Could you check a few things on this model? Use its own coordinates, in mm. Coordinates: 2 decimals unless noted, no trailing zeros. Order: outer loops, then holes, each group sorted by start corner. A loop starts at its lowest first (then second) coordinate and runs counter-clockwise, first axis right, second up. Notation, with made-up numbers: (82, 29) -> (113, 29) arc R8 cw to (113, 39) -> close; hole circle Ø5 at (-19.75, -9). An arc over 180 degrees is marked (long way). Use a Markdown table: item, result. Add a question column.
1) If we section it at C-C (y = 1.75): Write out the boundary of the cut face in (x, z), plus the area to 3 significant figures.
2) Will these pins go through, and if not, where does the flat tip stop? pin 1 Ø0.9 at (x, y) = (-95.5, 1) entering from +Z; pin 2 Ø1.5 at (x, y) = (-171.5, 1.5) entering from +Z; pin 3 Ø2.5 at (x, z) = (-47.5, -12) entering from -Y.
3) If we section it at D-D (x = -47.5): Write out the boundary of the cut face in (y, z), plus the area to 3 significant figures.
4) If we section it at A-A (x = -181.5): Write out the boundary of the cut face in (y, z), plus the area to 3 significant figures.
5) If I drill on L1, parallel to Z at x = -211.5, y = 2.3; L2, parallel to X at y = 0.8, z = -13; L3, parallel to X at y = 1.45, z = -9, over which ranges is the centre line in solid material (lowest first)? Write a range as [from, to].
6) If we section it at B-B (z = -22.5): Write out the boundary of the cut face in (x, y).
```python
from build123d import *

# Parameters (mm, degrees)
EXTRUDE_1_DEPTH     = 3
SKETCH_2_R          = 2
SKETCH_2_R_2        = 3
CUT_EXTRUDE_1_DEPTH = 10
FILLET_1_R          = 10
FILLET_2_R          = 2
FILLET_3_R          = 3


with BuildPart() as part:
    # 草图1 → 凸台-拉伸1 (new body)
    with BuildSketch(Plane(origin=(0, 0, 0), x_dir=(1, 0, 0), z_dir=(0, 1, 0))):
        with BuildLine():
            Line((-55, 0), (-40, 0))
            Line((-40, 0), (-40, 30))
            Line((-40, 30), (-113.286796564, 30))
            Line((-113.286796564, 30), (-143.786796564, 60.5))
            Line((-143.786796564, 60.5), (-209, 60.5))
            ThreePointArc((-209, 60.5), (-216.071067812, 57.571067812), (-219, 50.5))
            Line((-219, 50.5), (-219, 5.5))
            Line((-219, 5.5), (-204, 5.5))
            Line((-204, 5.5), (-204, 45.5))
            Line((-204, 45.5), (-150, 45.5))
            Line((-150, 45.5), (-119.5, 15))
            Line((-119.5, 15), (-55, 15))
            Line((-55, 15), (-55, 0))
        make_face()
    extrude(amount=EXTRUDE_1_DEPTH)

    # 草图2 → 切除-拉伸1 (cut)
    with BuildSketch(Plane(origin=(0, 3, 0), x_dir=(1, 0, 0), z_dir=(0, 1, 0))):
        with Locations(Location((-47.5, 12, 0), (0, 0, 270))):
            Circle(SKETCH_2_R)
        with Locations(Location((-211.5, 13, 0), (0, 0, 270))):
            Circle(SKETCH_2_R)
        with Locations(Location((-211.5, 28, 0), (0, 0, 270))):
            Circle(SKETCH_2_R)
        with Locations(Location((-209, 50.5, 0), (0, 0, 270))):
            Circle(SKETCH_2_R_2)
        with Locations(Location((-181.5, 53, 0), (0, 0, 270))):
            Circle(SKETCH_2_R)
        with Locations(Location((-122.5, 28, 0), (0, 0, 270))):
            Circle(SKETCH_2_R)
        with Locations(Location((-62.5, 22.5, 0), (0, 0, 270))):
            Circle(SKETCH_2_R)
    extrude(amount=-CUT_EXTRUDE_1_DEPTH, mode=Mode.SUBTRACT)

    # 圆角1
    fillet_1_edges = [part.edges().sort_by_distance(p)[0] for p in [
        (-119.5, 1.5, -15),
        (-150, 1.5, -45.5),
        (-143.786796564, 1.5, -60.5),
        (-113.286796564, 1.5, -30),
    ]]
    fillet(fillet_1_edges, radius=FILLET_1_R)

    # 圆角2
    fillet_2_edges = [part.edges().sort_by_distance(p)[0] for p in [
        (-40, 1.5, -30),
        (-55, 1.5, -15),
    ]]
    fillet(fillet_2_edges, radius=FILLET_2_R)

    # 圆角3
    fillet_3_edges = [part.edges().sort_by_distance(p)[0] for p in [
        (-204, 1.5, -45.5),
    ]]
    fillet(fillet_3_edges, radius=FILLET_3_R)


solid = part.part
```
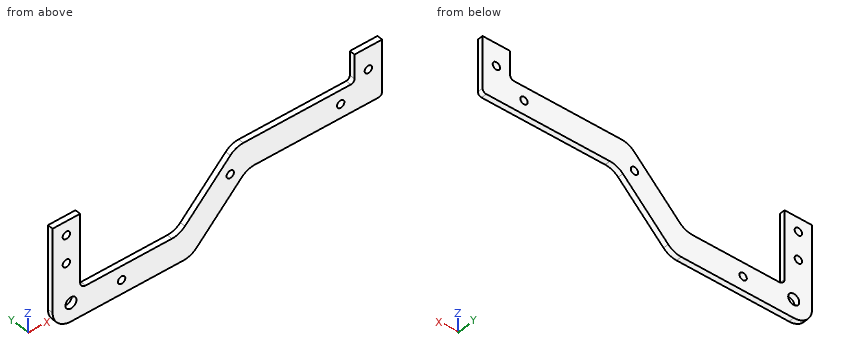
Answer sheet:
| question | item | result |
|---|---|---|
| 1 | outline | (-219, -50.5) arc R10 ccw to (-209, -60.5) -> (-147.93, -60.5) arc R10 ccw to (-140.86, -57.57) -> (-116.22, -32.93) arc R10 cw to (-109.14, -30) -> (-42, -30) arc R2 ccw to (-40, -28) -> (-40, 0) -> (-55, 0) -> (-55, -13) arc R2 cw to (-57, -15) -> (-115.36, -15) arc R10 ccw to (-122.43, -17.93) -> (-147.07, -42.57) arc R10 cw to (-154.14, -45.5) -> (-201, -45.5) arc R3 cw to (-204, -42.5) -> (-204, -5.5) -> (-219, -5.5) -> close; hole circle Ø4 at (-211.5, -28); hole circle Ø4 at (-211.5, -13); hole circle Ø6 at (-209, -50.5); hole circle Ø4 at (-181.5, -53); hole circle Ø4 at (-122.5, -28); hole circle Ø4 at (-62.5, -22.5); hole circle Ø4 at (-47.5, -12) |
| 1 | area | 3,580 mm2 |
| 2 | pin 1 | z = -15 |
| 2 | pin 2 | z = -45.5 |
| 2 | pin 3 | through |
| 3 | outline | (0, -30) -> (3, -30) -> (3, -14) -> (0, -14) -> close; (0, -10) -> (3, -10) -> (3, 0) -> (0, 0) -> close |
| 3 | area | 78.0 mm2 |
| 4 | outline | (0, -60.5) -> (3, -60.5) -> (3, -55) -> (0, -55) -> close; (0, -51) -> (3, -51) -> (3, -45.5) -> (0, -45.5) -> close |
| 4 | area | 33.0 mm2 |
| 5 | L1 | [-60.18, -52.16], [-48.84, -30], [-26, -15], [-11, -5.5] |
| 5 | L2 | [-219, -213.5], [-209.5, -204], [-55, -49.23], [-45.77, -40] |
| 5 | L3 | [-219, -204], [-55, -40] |
| 6 | outline | (-219, 0) -> (-204, 0) -> (-204, 3) -> (-219, 3) -> close; (-127, 0) -> (-64.5, 0) -> (-64.5, 3) -> (-127, 3) -> close; (-60.5, 0) -> (-40, 0) -> (-40, 3) -> (-60.5, 3) -> close |
